from build123d import *

# Parameters (mm, degrees)
BOSS_EXTRUDE1_DEPTH      = 6
BOSS_EXTRUDE1_DEPTH_BACK = 6
BOSS_EXTRUDE2_DEPTH      = 18
BOSS_EXTRUDE2_DEPTH_BACK = 18
SKETCH1_4_R              = 12.5


with BuildPart() as part:
    # Sketch1 → Boss-Extrude1 (new, two sides: drawn at the far end of the back side and taken through both)
    with BuildSketch(Plane.XY.offset(-BOSS_EXTRUDE1_DEPTH_BACK)):
        with BuildLine():
            ThreePointArc((8.486454979, 38.065470993), (-9.029705239, 51.210003157), (-20.993816965, 32.86730365))
            ThreePointArc((-20.993816965, 32.86730365), (6.772278929, -38.407502367), (8.486454979, 38.065470993))
        make_face()
        with BuildLine():
            Line((-2, 6.2), (2, 6.2))
            Line((2, 6.2), (2, 4.8))
            ThreePointArc((2, 4.8), (0, -5.2), (-2, 4.8))
            Line((-2, 4.8), (-2, 6.2))
        make_face(mode=Mode.SUBTRACT)
    extrude(amount=BOSS_EXTRUDE1_DEPTH + BOSS_EXTRUDE1_DEPTH_BACK)

    # Sketch1<4> → Boss-Extrude2 (add, two sides: drawn at the far end of the back side and taken through both)
    with BuildSketch(Plane.XY.offset(-BOSS_EXTRUDE2_DEPTH_BACK)):
        Circle(SKETCH1_4_R)
        with BuildLine():
            Line((-2, 4.8), (-2, 6.2))
            Line((-2, 6.2), (2, 6.2))
            Line((2, 6.2), (2, 4.8))
            ThreePointArc((2, 4.8), (4.326661531, 2.88444102), (5.2, 0))
            ThreePointArc((5.2, 0), (-2.88444102, -4.326661531), (-2, 4.8))
        make_face(mode=Mode.SUBTRACT)
    extrude(amount=BOSS_EXTRUDE2_DEPTH + BOSS_EXTRUDE2_DEPTH_BACK)


solid = part.part
The model under review builds one solid part; all positions refer to its coordinate system, in mm. A direction names the side the tool comes from. Give positions to 0.01 mm unless a question says otherwise; leave off trailing zeros. Write each loop counter-clockwise with the first axis right and the second up, starting at its lowest first coordinate (ties: lowest second). Pieces come first, ordered by that corner, then holes.
1. Add section C-C, the plane y = 8.5. Write out the cut boundary in (x, z).
2. Tool access review of faces 1 (the cylindrical face through (11.923, 3.755, -12.084)), 2 (the cylindrical face through (11.923, 3.755, 11.916)), 3 (the flat face through (-0.2, -5.4, 18)): name each direction out of +Z, -Z, +X, -X, +Y, -Y from which nothing blocks a thin tool from reaching the whole face with its end or side.
3. Add section D-D, the plane z = -2.5. Write out the cut boundary in (x, y), plus the area to 3 significant figures.
4. Draft analysis for pull direction X (two halves, no side actions). For faces 4 (the cylindrical face through (-8.691, 51.266, -0.084)), 5 (the flat face through (-0.2, -5.4, -18)), 6 (the flat face through (0, 6.2, 0)), state which applies: +X half, -X half, draft (parallel to the pull), parting line (faces both ways), or undercut.
5. For P1, Ø1.5, axis at y = 5.5, z = -1, coming from the -X side; P2, Ø8, axis at x = -2.5, y = 27, coming from the -Z side; P3, Ø23.5, axis at x = -15, y = 0.5, coming from the -Z side; P4, Ø4, axis at y = -21, z = -4.5, coming from the +X side, all flat-tipped, find the tip position at first contact; note any pin that passes through.
6. Wall thickness on L1, parallel to X at y = 0, z = -14.5; L2, parallel to Y at x = 0, z = 10; L3, parallel to Z at x = -30.5, y = -15: over which ranges is each line inside the solid? List them lowest first.
7. Add section A-A, the plane x = 0. Write out the cut boundary in (y, z).
8. Add section B-B, the plane z = -9. Write out the cut boundary in (x, y).
Worked answers:
1. outline: (-38.06, -6) - (-9.17, -6) - (-9.17, -18) - (9.17, -18) - (9.17, -6) - (38.06, -6) - (38.06, 6) - (9.17, 6) - (9.17, 18) - (-9.17, 18) - (-9.17, 6) - (-38.06, 6) - close
2. face 1: -Z
2. face 2: +Z
2. face 3: +Z, +X, -X, +Y, -Y
3. outline: (-20.99, 32.87) arc R39 ccw (long way) to (8.49, 38.07) arc R15 ccw (long way) to start; hole (-2, 4.8) arc R5.2 ccw (long way) to (2, 4.8) - (2, 6.2) - (-2, 6.2) - close
3. area: 5,010 mm2
4. face 4: parting line
4. face 5: draft
4. face 6: undercut
5. P1: stops at x = -38.71
5. P2: stops at z = -6
5. P3: stops at z = -18
5. P4: stops at x = 34.06
6. L1: x = -12.5 to -5.2, 5.2 to 12.5
6. L2: y = -12.5 to -5.2, 6.2 to 12.5
6. L3: z = -6 to 6
7. outline: (-39, -6) - (-12.5, -6) - (-12.5, -18) - (-5.2, -18) - (-5.2, 18) - (-12.5, 18) - (-12.5, 6) - (-39, 6) - close; (6.2, -18) - (12.5, -18) - (12.5, -6) - (49.99, -6) - (49.99, 6) - (12.5, 6) - (12.5, 18) - (6.2, 18) - close
8. outline: circle Ø25 at (0, 0); hole (-2, 4.8) arc R5.2 ccw (long way) to (2, 4.8) - (2, 6.2) - (-2, 6.2) - close
